Autodesk Fusion 360 part; units mm, degrees
sketch "Skizze1" plane through (0, 0, 0) normal (0, 0, 1) x (1, 0, 0)
  circle A0 centre (0, 0) radius 7.65
  line L0 (15, -10) -> (-15, -10)
  line L1 (-15, -10) -> (-15, 15)
  line L2 (-15, 15) -> (15, 15)
  line L3 (15, 15) -> (15, -10)
  line L4 (0, 0) -> (0, -10)
  line L5 (0, -10) -> (-0.5, -10)
  line L6 (-0.5, -10) -> (0.5, -10)
  line L7 (0.5, -10) -> (0.5, -7.3)
  line L8 (0.5, -7.3) -> (-0.5, -7.3)
  line L9 (-0.5, -7.3) -> (-0.5, -10)
  circle A1 centre (0, 0) radius 15
  dimension "d1" = 15.3
  dimension "d4" = 15
  dimension "d5" = 10
  dimension "d6" = 15
  dimension "d7" = 25
extrude "Extrusion1" add sketch "Skizze1" along normal blind 50 contours A0 L0 L7 L9 A1 | L0 L3 A1 | L2 L3 A1
sketch "Skizze2" plane through (15, 0, 0) normal (1, 0, 0) x (0, 1, 0)
  line L0 (-10, 0) -> (15, 0)
  line L1 (15, 0) -> (15, 50)
  line L2 (15, 50) -> (-10, 50)
  line L3 (-10, 50) -> (-10, 0)
  line L4 (-10, 25) -> (15, 25)
  circle A0 centre (0, 25) radius 4.15
  line L5 (0, 25) -> (0, 42.5)
  line L6 (0, 25) -> (0, 7.5)
  circle A1 centre (0, 42.5) radius 4.15
  circle A2 centre (0, 7.5) radius 4.15
  dimension "d10" = 8.3
  dimension "d11" = 10
  dimension "d22" = 17.5
  dimension "d23" = 8.3
  dimension "d24" = 8.3
  dimension "d25" = 17.5
extrude "Extrusion2" cut sketch "Skizze2" against normal blind 6 contours A2 | A1 | L4 A0 L5 | L4 A0 L6 | L4 A0 L6 | L4 A0 L5
extrude "Extrusion4" add 1 faces at (15, 11.3833, 25) along direction (1, 0, 0) blind 10
sketch "Skizze3" plane through (0, 15, 0) normal (0, 1, 0) x (-1, 0, 0)
  line L0 (-25, 0) -> (0, 0)
  line L1 (0, 50) -> (-25, 50)
  line L2 (-25, 25) -> (-18, 25)
  line L3 (-18, 25) -> (-18, 20.25)
  line L4 (-18, 25) -> (-18, 29.75)
  circle A0 centre (-18, 29.75) radius 1.5
  circle A1 centre (-18, 20.25) radius 1.5
  line L5 (0, 0) -> (0, 50)
  line L6 (-25, 50) -> (-25, 0)
  dimension "d15" = 7
  dimension "d16" = 4.75
  dimension "d17" = 4.75
  dimension "d18" = 3
  dimension "d19" = 3
extrude "Extrusion3" cut sketch "Skizze3" against normal blind 5 contours A0 | A1
Design review of the part built by this model. Coordinates are the model's own, in mm. A direction names the side the tool comes from. Coordinates: 2 decimals unless noted, no trailing zeros. Write each loop counter-clockwise with the first axis right and the second up, starting at its lowest first coordinate (ties: lowest second). Pieces come first, ordered by that corner, then holes.
1) Add section A-A (x = 21). Write out the cut boundary in (y, z).
2) Add section D-D (y = -4.75). Write out the cut boundary in (x, z), plus the area to 3 significant figures.
3) Add section C-C (z = 20.25). Write out the cut boundary in (x, y), plus the area to 4 significant figures.
4) Machinability: for faces 4 (the flat face through (9, 3, 0)), 5 (the flat face through (-0.5, -9, 25)), 6 (the cylindrical face through (-13.79, 5.9, 24.65)), 7 (the flat face through (9, 0, 43)), 8 (the cylindrical face through (19.11, 12.54, 21.26)), which of the approach directions +Z, -Z, +X, -X, +Y, -Y give a long, thin tool a straight path to every point of the face, cutting with its end or side? Answer none if there is none.
5) Insertion check: pin 1 (0.9 mm diameter, centred on x = 18.5, z = 20, fed in from +Y); pin 2 (14 mm diameter, centred on x = 0, y = 0, fed in from +Z); pin 3 (2.5 mm diameter, centred on y = -9.5, z = 30, fed in from -X). Each pin has a flat end and moves straight along its axis. Give the tip position at first contact, or say it passes through.
6) To check wall thickness, follow L1, parallel to Z at x = 19.25, y = 0; L2, parallel to Z at x = 18, y = 11; L3, parallel to Z at x = 21.5, y = -1.5. State the ranges of each line that lie inside material, in increasing order.
7) Add section B-B (y = 2). Write out the cut boundary in (x, z), plus the area to 3 significant figures.
8) Mouldability with a two-part tool opening along X and no side actions: class faces 1 (the flat face through (9, 0, 25)), 2 (the flat face through (18, 10, 20)), 3 (the flat face through (-6, -10, 25)) as +X half, -X half, draft (parallel to the pull), parting line (faces both ways), or undercut.
Check result:
1. outline: (-10, 0) - (15, 0) - (15, 50) - (-10, 50) - close; hole circle Ø8.3 at (0, 7.5); hole circle Ø8.3 at (0, 25); hole circle Ø8.3 at (0, 42.5)
2. outline: (-14.23, 0) - (-6, 0) - (-6, 50) - (-14.23, 50) - close; (6, 0) - (25, 0) - (25, 50) - (6, 50) - close
2. area: 1,360 mm2
3. outline: (-11.18, -10) - (-0.5, -10) - (-0.5, -7.63) arc R7.65 cw (long way) to (0.5, -7.63) - (0.5, -10) - (25, -10) - (25, 15) - (19.5, 15) - (19.5, 10) - (16.5, 10) - (16.5, 15) - (0, 15) arc R15 ccw to start
3. area: 738.5 mm2
4. face 4: -Z, +X, -X, +Y, -Y
4. face 5: +Z, -Z, -Y
4. face 6: +Z, -Z, -X
4. face 7: +X
4. face 8: +Y
5. pin 1: stops at y = 10
5. pin 2: passes through
5. pin 3: stops at x = -12.53
6. L1: z = 0 to 3.35, 11.65 to 20.85, 29.15 to 38.35, 46.65 to 50
6. L2: z = 0 to 18.75, 21.75 to 28.25, 31.25 to 50
6. L3: z = 0 to 3.63, 11.37 to 21.13, 28.87 to 38.63, 46.37 to 50
7. outline: (-14.87, 0) - (-7.38, 0) - (-7.38, 50) - (-14.87, 50) - close; (7.38, 0) - (25, 0) - (25, 3.86) - (9, 3.86) - (9, 11.14) - (25, 11.14) - (25, 21.36) - (9, 21.36) - (9, 28.64) - (25, 28.64) - (25, 38.86) - (9, 38.86) - (9, 46.14) - (25, 46.14) - (25, 50) - (7.38, 50) - close
7. area: 906 mm2
8. face 1: +X half
8. face 2: undercut
8. face 3: draft
